Source: CAD feature listing. Evaluate the final solid. Frame: model axes, mm. Face numbers are marked on the shaded views. A direction names the side the tool comes from. Round coordinates to 2 decimals unless told otherwise and drop trailing zeros. Loops run counter-clockwise (first coordinate to the right, second up) from the corner with the lowest first, then second, coordinate; pieces in that order, holes last. Notation, with made-up numbers: (46, 79) -> (52, 79) arc R26 cw to (52, 111) -> close; hole circle Ø11 at (31.25, 64.5). An arc over 180 degrees is marked (long way). Return JSON: item names as keys, results as strings. Group by question number.
```python
from build123d import *

# Parameters (mm, degrees)
SKETCH1_W                                    = 30
SKETCH1_H                                    = 25
BOSS_EXTRUDE1_DEPTH                          = 10
FILLET1_R                                    = 5
CBORE_FOR_M6_HEX_SOCKET_HEAD_CAP_SCR_2_COUNT = 2
CBORE_FOR_M6_HEX_SOCKET_HEAD_CAP_SCR_2_PITCH = 12
CHAMFER1_SIZE                                = 2


with BuildPart() as part:
    # Sketch1 → Boss-Extrude1 (new body)
    with BuildSketch(Plane(origin=(0, 0, 0), x_dir=(1, 0, 0), z_dir=(0, 1, 0))):
        Rectangle(SKETCH1_W, SKETCH1_H)
    extrude(amount=BOSS_EXTRUDE1_DEPTH)

    # Fillet1
    fillet1_edges = [part.edges().sort_by_distance(p)[0] for p in [
        (-15, 5, -12.5),
        (-15, 5, 12.5),
    ]]
    fillet(fillet1_edges, radius=FILLET1_R)

    # Sketch3 → CBORE for M6 Hex Socket Head Cap Screw1 (revolve, cut)
    with BuildSketch(Plane(origin=(-5, 10, -6), x_dir=(0, 0, 1), z_dir=(1, 0, 0))):
        Polygon((0, 0), (0, 10), (3.325, 10), (3.3, 9.975), (3.3, 6.4), (5.5, 6.4), (5.5, 0.025), (5.525, 0), align=None)
    cbore_for_m6_hex_socket_head_cap_screw1 = revolve(axis=Axis((-5, 16.35, -6), (0, -1, 0)), mode=Mode.SUBTRACT)

    # CBORE for M6 Hex Socket Head Cap Scr 2: CBORE for M6 Hex Socket Head Cap Screw1 ×2
    with Locations(*[(0, 0, i * CBORE_FOR_M6_HEX_SOCKET_HEAD_CAP_SCR_2_PITCH) for i in range(1, CBORE_FOR_M6_HEX_SOCKET_HEAD_CAP_SCR_2_COUNT)]):
        add(cbore_for_m6_hex_socket_head_cap_screw1, mode=Mode.SUBTRACT)

    # Sketch5 → M6 Tapped Hole1 (revolve, cut)
    with BuildSketch(Plane(origin=(5.715161352, 0, 0), x_dir=(0, 0, -1), z_dir=(1, 0, 0))):
        Polygon((0, 0), (0, 10), (3.025, 10), (2.5, 9.475), (2.5, 0.525), (3.025, 0), align=None)
    revolve(axis=Axis((5.715161352, -6.35, 0), (0, 1, 0)), mode=Mode.SUBTRACT)

    # Chamfer1
    chamfer1_edges = [part.edges().sort_by_distance(p)[0] for p in [
        (15, 5, -12.5),
        (15, 5, 12.5),
    ]]
    chamfer(chamfer1_edges, length=CHAMFER1_SIZE)


solid = part.part
```
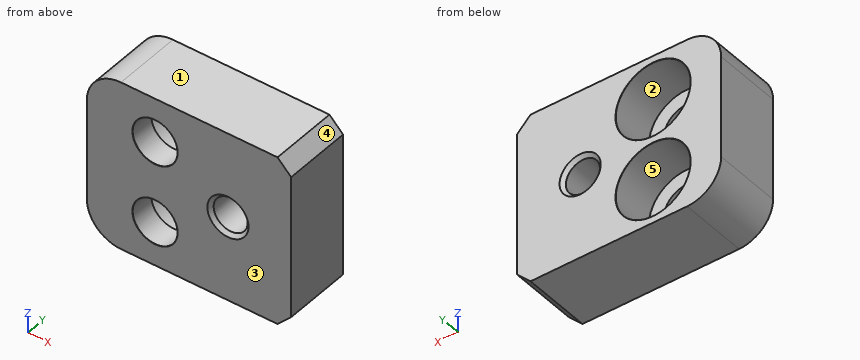
(1) Set-up query: the marked faces 1 and 2. Return all of +Z, -Z, +X, -X, +Y, -Y with unobstructed straight access to the full face (end or side cutting, diameter ignored); none if empty.
(2) Cut plane A-A (z = 0). Return loops of the section in (x, y) (3 decimals), and give its area (3 significant figures).
(3) Cut plane C-C (y = 8.5). Return loops of the section in (x, z), and give its area (3 significant figures).
(4) Ray query, line 1 (Z direction, x = -5, y = 6.25); line 2 (Z direction, x = -5, y = 1); line 3 (X direction, y = 7, z = -6). Return the intervals inside material, ascending.
(5) Cut plane D-D (z = -6). Return loops of the section in (x, y) (3 decimals).
(6) Mould query, pull axis Z, two halves, no side actions, for the marked faces 3, 4 and 5. Classes: released by +Z, released by -Z, zero draft, split by the parting line, or undercut.
(7) Cut plane B-B (x = -5). Return loops of the section in (y, z) (3 decimals), and give its area (3 significant figures).
(8) Pin query (flat end, axial travel): pin 1 (4 mm diameter, centred on x = -5, z = -6, fed in from +Y); pin 2 (9 mm diameter, centred on x = -4, z = -3.5, fed in from +Y); pin 3 (10.5 mm diameter, centred on x = -5, z = 6, fed in from +Y). Return the tip coordinate at first contact, or that it passes through.
Answers follow:
{
 "1": {"face 1": "+Z, +X, -X, +Y, -Y", "face 2": "+Y"},
 "2": {"outline": "(-15, 0) -> (2.69, 0) -> (3.215, 0.525) -> (3.215, 9.475) -> (2.69, 10) -> (-15, 10) -> close; (8.215, 0.525) -> (8.74, 0) -> (15, 0) -> (15, 10) -> (8.74, 10) -> (8.215, 9.475) -> close", "area": "249 mm^2"},
 "3": {"outline": "(-15, -7.5) arc R5 ccw to (-10, -12.5) -> (13, -12.5) -> (15, -10.5) -> (15, 10.5) -> (13, 12.5) -> (-10, 12.5) arc R5 ccw to (-15, 7.5) -> close; hole circle Ø11 at (-5, -6); hole circle Ø11 at (-5, 6); hole circle Ø5 at (5.72, 0)", "area": "526 mm^2"},
 "4": {"line 1": "-12.5 to -11.5, -0.5 to 0.5, 11.5 to 12.5", "line 2": "-12.5 to -9.3, -2.7 to 2.7, 9.3 to 12.5", "line 3": "-15 to -10.5, 0.5 to 15"},
 "5": {"outline": "(-15, 0) -> (-8.325, 0) -> (-8.3, 0.025) -> (-8.3, 3.6) -> (-10.5, 3.6) -> (-10.5, 9.975) -> (-10.525, 10) -> (-15, 10) -> close; (-1.7, 0.025) -> (-1.675, 0) -> (15, 0) -> (15, 10) -> (0.525, 10) -> (0.5, 9.975) -> (0.5, 3.6) -> (-1.7, 3.6) -> close"},
 "6": {"face 3": "zero draft", "face 4": "released by +Z", "face 5": "undercut"},
 "7": {"outline": "(0, -12.5) -> (10, -12.5) -> (10, -11.525) -> (9.975, -11.5) -> (3.6, -11.5) -> (3.6, -9.3) -> (0.025, -9.3) -> (0, -9.325) -> close; (0, -2.675) -> (0.025, -2.7) -> (3.6, -2.7) -> (3.6, -0.5) -> (9.975, -0.5) -> (10, -0.475) -> (10, 0.475) -> (9.975, 0.5) -> (3.6, 0.5) -> (3.6, 2.7) -> (0.025, 2.7) -> (0, 2.675) -> close; (0, 9.325) -> (0.025, 9.3) -> (3.6, 9.3) -> (3.6, 11.5) -> (9.975, 11.5) -> (10, 11.525) -> (10, 12.5) -> (0, 12.5) -> close", "area": "61.7 mm^2"},
 "8": {"pin 1": "through", "pin 2": "y = 10", "pin 3": "y = 3.6"}
}
